from build123d import *

# Parameters (mm, degrees)
F1_START = 15
F1_DEPTH = 15
F2_DEPTH = 25


with BuildPart() as f1:
    # F0 (on Top) → F1 (new body)
    with BuildSketch(Plane.XY.offset(F1_START)):
        Polygon((28.5, -14), (28.5, 14), (-28.5, 14), (-28.5, 11.3388504833), (-28.5, -11.4388540387), (-28.5, -14), align=None)
        Polygon((-28.5, -11.4388540387), (-28.5, 11.3388504833), (-33.5, 10.6412195601), (-33.5, -10.740224272), align=None)
        Polygon((-33.5, -10.740224272), (-33.5, 10.6412195601), (-38.5, 9.9435886368), (-38.5, -10.0415945053), align=None)
    extrude(amount=F1_DEPTH)

    # F0 (on Top) → F2 (join)
    with BuildSketch(Plane.XY):
        Polygon((-38.5, 9.9435886368), (-33.5, 10.6412195601), (-33.5, 15.6896538624), (-43.5, 14.2943920159), (-43.5, -14.3915371656), (-33.5, -15.788796699), (-33.5, -10.740224272), (-38.5, -10.0415945053), align=None)
        Polygon((-28.5, 14), (28.5, 14), (28.5, -14), (-28.5, -14), (-28.5, -11.4388540387), (-33.5, -10.740224272), (-33.5, -15.788796699), (-33.5, -19), (33.5, -19), (33.5, 19), (-33.5, 19), (-33.5, 15.6896538624), (-33.5, 10.6412195601), (-28.5, 11.3388504833), align=None)
    extrude(amount=F2_DEPTH)


solid = f1.part
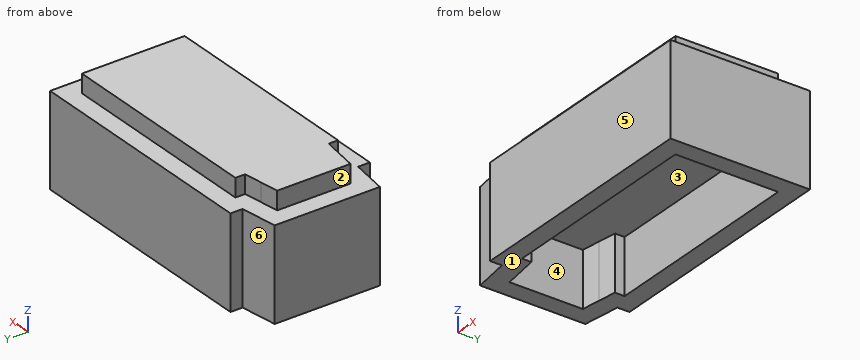
Here's how the part is built. I have some questions about the finished solid (model axes, mm). Face numbers are marked on the shaded views. A direction names the side the tool comes from. Give positions to 0.01 mm unless a question says otherwise; leave off trailing zeros. Order: outer loops, then holes, each group sorted by start corner. A loop starts at its lowest first (then second) coordinate and runs counter-clockwise, first axis right, second up. Notation, with made-up numbers: (24, 30.25) -> (60, 30.25) arc R15 ccw to (60, 45.25) -> close; hole circle Ø7 at (45, 12.25). An arc over 180 degrees is marked (long way). One line per item, written item: value. Start each with the question number.
1. For the marked faces 1, 2 and 3, which set-ups out of +Z, -Z, +X, -X, +Y, -Y let a thin tool reach every point of the face, with its end or its side?
2. Will these pins go through, and if not, where does the flat tip stop? pin 1 Ø1.5 at (y, z) = (3, 27.5) entering from -X; pin 2 Ø10 at (x, y) = (10, 7.5) entering from -Z; pin 3 Ø1.5 at (x, z) = (-7.5, 27.5) entering from -Y.
3. We'd pull the mould along Y, two halves only. Please class the marked faces 4, 5 and 6: released by +Y, released by -Y, zero draft, split by the parting line, or undercut.
4. I need wall thicknesses on probe 1 along X at (y, z) = (-3, 3.5); probe 2 along Y at (x, z) = (-11.5, 4.75); probe 3 along Z at (x, y) = (25, -12). Which ranges of each line are inside material? Lowest first, please. Write a range as from..to.
5. Imagine slicing it at C-C, the plane y = 13. List the corners of the cut face in (x, z) for me, plus the area to 4 significant figures.
6. Imagine slicing it at B-B, the plane x = -27.5. List the corners of the cut face in (y, z) for me, plus the area to 3 significant figures.
7. Imagine slicing it at A-A, the plane z = 27.5. List the corners of the cut face in (x, y) for me, plus the area to 3 significant figures.
8. Imagine slicing it at D-D, the plane z = 7.75. List the corners of the cut face in (x, y) for me, plus the area to 3 significant figures.
Values follow:
1. face 1: -Z, +X, -X, +Y, -Y
1. face 2: +Z, -X, +Y, -Y
1. face 3: -Z
2. pin 1: stops at x = -38.5
2. pin 2: stops at z = 15
2. pin 3: stops at y = -14
3. face 4: undercut
3. face 5: released by -Y
3. face 6: released by +Y
4. probe 1: x = -43.5..-38.5, 28.5..33.5
4. probe 2: y = -19..-14, 14..19
4. probe 3: z = 15..30
5. outline: (-43.5, 0) -> (-28.5, 0) -> (-28.5, 15) -> (28.5, 15) -> (28.5, 0) -> (33.5, 0) -> (33.5, 25) -> (28.5, 25) -> (28.5, 30) -> (-28.5, 30) -> (-28.5, 25) -> (-43.5, 25) -> close
5. area: 1,355 mm2
6. outline: (-19, 0) -> (-14, 0) -> (-14, 15) -> (14, 15) -> (14, 0) -> (19, 0) -> (19, 25) -> (14, 25) -> (14, 30) -> (-14, 30) -> (-14, 25) -> (-19, 25) -> close
6. area: 670 mm2
7. outline: (-38.5, -10.04) -> (-28.5, -11.44) -> (-28.5, -14) -> (28.5, -14) -> (28.5, 14) -> (-28.5, 14) -> (-28.5, 11.34) -> (-38.5, 9.94) -> close
7. area: 1,810 mm2
8. outline: (-43.5, -14.39) -> (-33.5, -15.79) -> (-33.5, -19) -> (33.5, -19) -> (33.5, 19) -> (-33.5, 19) -> (-33.5, 15.69) -> (-43.5, 14.29) -> close; hole (-38.5, -10.04) -> (-28.5, -11.44) -> (-28.5, -14) -> (28.5, -14) -> (28.5, 14) -> (-28.5, 14) -> (-28.5, 11.34) -> (-38.5, 9.94) -> close
8. area: 1,040 mm2
